Design review of the part built by this model. Coordinates are the model's own, in mm. A direction names the side the tool comes from. Coordinates: 2 decimals unless noted, no trailing zeros. Loops run counter-clockwise (first coordinate to the right, second up) from the corner with the lowest first, then second, coordinate; pieces in that order, holes last. Notation, with made-up numbers: (77.25, 72) -> (112.25, 72) arc R22 ccw to (112.25, 80) -> close; hole circle Ø8 at (85.5, -13). An arc over 180 degrees is marked (long way). Use a Markdown table: item, result. Add a question column.
Q1. Take a section at B-B on y = 80. Write out the cut boundary in (x, z), plus the area to 3 significant figures.
Q2. Take a section at C-C on z = 2.75. Write out the cut boundary in (x, y).
Q3. Take a section at D-D on x = 3.5. Write out the cut boundary in (y, z).
Q4. For faces 1 (the face through (59, 60, 5)), 2 (the face through (115, 5, 5)), list the 3-axis set-ups (+Z, -Z, +X, -X, +Y, -Y) from which the entire face can be reached by the end or side of a thin tool; tool diameter is ignored.
Q5. Clearance check with flat-ended pins moving along their axes: pin 1 Ø3 at (y, z) = (74, 7) entering from +X; pin 2 Ø4 at (x, z) = (38, 3) entering from +Y (3 decimals). State where each tip first meets the part, or that it passes through.
Q6. Take a section at A-A on x = -40. Write out the cut boundary in (y, z).
Q7. For probe 1 along X at (y, z) = (53, 9.25); probe 2 along X at (y, z) = (43.5, 8); probe 3 along X at (y, z) = (65, 5), list the stretches that pass through material, from the lowest coordinate up.
Q8. Draft analysis for pull direction Y (two halves, no side actions). For faces 3 (the face through (54, 0, 5)), 4 (the face through (23, 67, 0)), 5 (the face through (-33.41, 41.286, 4.93)), state which applies: pulls with the +Y half, pulls with the -Y half, needs draft (parallel to the pull), parting line crosses it, or undercut.
from build123d import *
from OCP.BRepFilletAPI import BRepFilletAPI_MakeChamfer

# Parameters (mm, degrees)
ESQUISSE1_R        = 23.5
ESQUISSE1_W        = 80
ESQUISSE1_H        = 40
BOSS_EXTRU_1_DEPTH = 10
CHANFREIN1_SIZE    = 10
CHANFREIN1_SIZE2   = 12.608056975


with BuildPart() as part:
    # Esquisse1 → Boss.-Extru.1 (new body)
    with BuildSketch(Plane.XY):
        with BuildLine():
            Line((0, 0), (120, 0))
            Line((120, 0), (120, 80))
            Line((120, 80), (-20.100018314, 106.944225709))
            ThreePointArc((-20.100018314, 106.944225709), (-69.345781346, 78.675628662), (-48.678780146, 25.787692258))
            Line((-48.678780146, 25.787692258), (0, 0))
        make_face()
        with Locations((-28.315442857, 64.227053523)):
            Circle(ESQUISSE1_R, mode=Mode.SUBTRACT)
        with Locations((60, 40)):
            Rectangle(ESQUISSE1_W, ESQUISSE1_H, mode=Mode.SUBTRACT)
    extrude(amount=BOSS_EXTRU_1_DEPTH)

    # Chanfrein1: one chamfer whose edges measure the first distance from different faces: ONE call of the kernel's chamfer builder (chamfer() names one face for all edges)
    chanfrein1_edges_1 = [part.edges().sort_by_distance(p)[0] for p in [
        (120, 80, 5),
    ]]
    chanfrein1_side_1 = [part.faces().sort_by_distance(p)[0] for p in [
        (120, 40, 5),
    ]]
    chanfrein1_edges_2 = [part.edges().sort_by_distance(p)[0] for p in [
        (120, 0, 5),
    ]]
    chanfrein1 = BRepFilletAPI_MakeChamfer(part.part.solid().wrapped)
    for e in chanfrein1_edges_1:
        chanfrein1.Add(CHANFREIN1_SIZE, CHANFREIN1_SIZE2, e.wrapped, chanfrein1_side_1[0].wrapped)  # the first distance lies on this face
    for e in chanfrein1_edges_2:
        chanfrein1.Add(CHANFREIN1_SIZE, e.wrapped)
    add(Compound.cast(chanfrein1.Shape()), mode=Mode.REPLACE)


solid = part.part
Answer list:
| question | item | result |
|---|---|---|
| 1 | outline | (-68.86, 0) -> (-45.74, 0) -> (-45.74, 10) -> (-68.86, 10) -> close; (-10.9, 0) -> (110, 0) -> (110, 10) -> (-10.9, 10) -> close |
| 1 | area | 1,440 mm² |
| 2 | outline | (-48.68, 25.79) -> (0, 0) -> (110, 0) -> (120, 10) -> (120, 70) -> (107.62, 82.38) -> (-20.1, 106.94) arc R43.5 ccw to start; hole circle Ø47 at (-28.32, 64.23); hole (20, 20) -> (100, 20) -> (100, 60) -> (20, 60) -> close |
| 3 | outline | (0, 0) -> (102.41, 0) -> (102.41, 10) -> (0, 10) -> close |
| 4 | face 1 | +Z, -Z |
| 4 | face 2 | +Z, -Z, +X, -Y |
| 5 | pin 1 | x = 117.5 |
| 5 | pin 2 | y = 96.155 |
| 6 | outline | (21.19, 0) -> (43.84, 0) -> (43.84, 10) -> (21.19, 10) -> close; (84.62, 0) -> (106.13, 0) -> (106.13, 10) -> (84.62, 10) -> close |
| 7 | probe 1 | -70.34 to -48.96, -7.67 to 20, 100 to 120 |
| 7 | probe 2 | -66.56 to -39.39, -17.24 to 20, 100 to 120 |
| 7 | probe 3 | -71.81 to -51.8, -4.83 to 120 |
| 8 | face 3 | pulls with the -Y half |
| 8 | face 4 | needs draft |
| 8 | face 5 | undercut |
